For this review, use the dimensioned drawing (mm, ordinates from the lowest corner) and the shaded views. A direction names the side the tool comes from. Coordinates: 2 decimals unless noted, no trailing zeros. Order: outer loops, then holes, each group sorted by start corner. A loop starts at its lowest first (then second) coordinate and runs counter-clockwise, first axis right, second up. Notation, with made-up numbers: M -2,63 L 3,63 A24 cw 3,80 Z; hole C 70,50.25 d10. An arc over 180 degrees is marked long. Use CSV: the item, a comma, the result in double quotes.
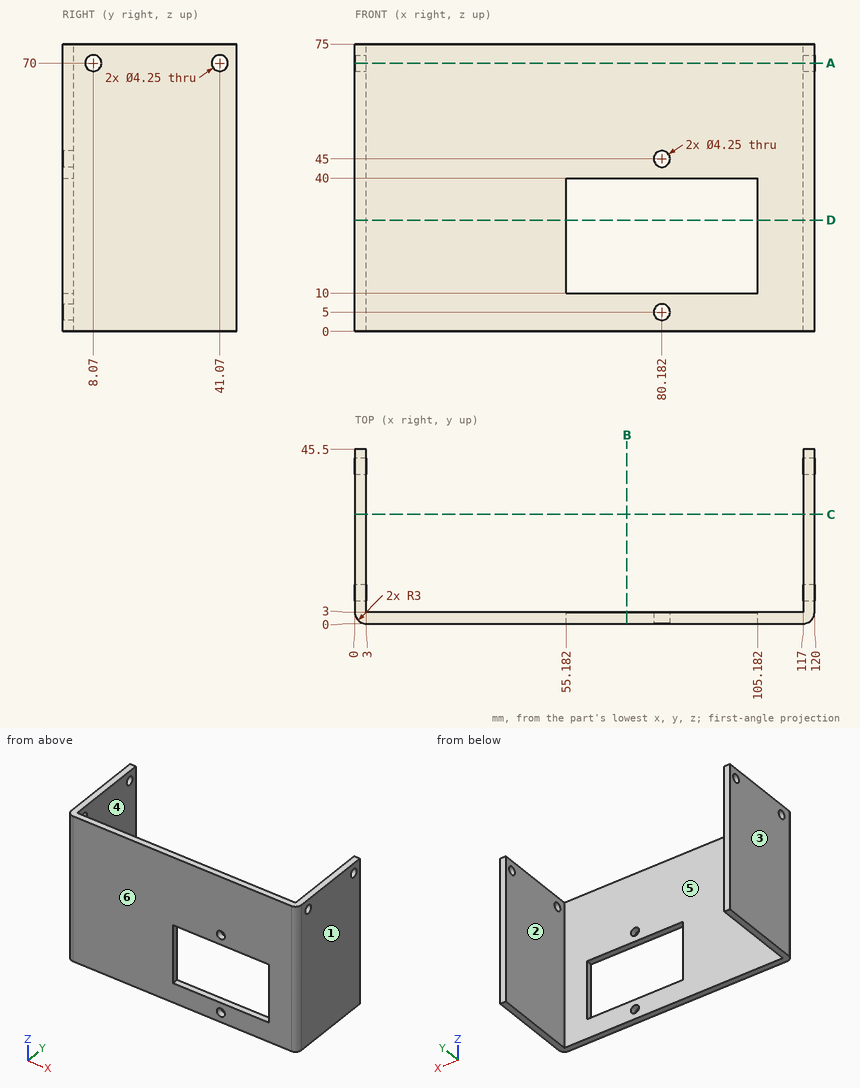
Item 1: Add section A-A on z = 70. State the section outline as (x, y) points (3 decimals), and give its area (3 significant figures).
Solutions:
outline,"M 0,3 A3 ccw 3,0 L 117,0 A3 ccw 120,3 L 120,5.945 L 117,5.945 L 117,3 L 3,3 L 3,5.945 L 0,5.945 Z; M 0,10.195 L 3,10.195 L 3,38.945 L 0,38.945 Z; M 0,43.195 L 3,43.195 L 3,45.5 L 0,45.5 Z; M 117,10.195 L 120,10.195 L 120,38.945 L 117,38.945 Z; M 117,43.195 L 120,43.195 L 120,45.5 L 117,45.5 Z"
area,"560 mm^2"
Item 2: To check wall thickness, follow line 1 along X through (y, z) = (43, 49.5); line 2 along Z through (x, y) = (70, 2); line 3 along Y through (x, z) = (14, 25.5). State the ranges of each line that lie inside material, in increasing order. Write a range as [from, to].
Solutions:
line 1,"[0, 3], [117, 120]"
line 2,"[0, 10], [40, 75]"
line 3,"[0, 3]"
Item 3: Clearance check with a flat-ended pin moving along its axis: pin 1 Ø3 at (x, z) = (63, 61.5) entering from +Y. State where the tip first meets the part, or that it passes through.
Solutions:
pin 1,"y = 3"
Item 4: For the marked faces 1 and 2, list the 3-axis set-ups (+Z, -Z, +X, -X, +Y, -Y) from which the entire face can be reached by the end or side of a thin tool; tool diameter is ignored.
Solutions:
face 1,"+Z, -Z, +X, +Y, -Y"
face 2,"+Z, -Z, +Y"
Item 5: Add section D-D on z = 29. State the section outline as (x, y) points, and give its area (3 significant figures).
Solutions:
outline,"M 0,3 A3 ccw 3,0 L 55.18,0 L 55.18,3 L 3,3 L 3,45.5 L 0,45.5 Z; M 105.18,0 L 117,0 A3 ccw 120,3 L 120,45.5 L 117,45.5 L 117,3 L 105.18,3 Z"
area,"461 mm^2"
Item 6: Add section C-C on y = 28.5. State the section outline as (x, z) points, and give its area (3 significant figures).
Solutions:
outline,"M 0,0 L 3,0 L 3,75 L 0,75 Z; M 117,0 L 120,0 L 120,75 L 117,75 Z"
area,"450 mm^2"
Item 7: Draft analysis for pull direction X (two halves, no side actions). For the marked faces 3, 4, 5 and 6, state which applies: released by +X, released by -X, zero draft, split by the parting line, or undercut.
Solutions:
face 3,"released by -X"
face 4,"undercut"
face 5,"undercut"
face 6,"zero draft"
Item 8: Add section B-B on x = 71. State the section outline as (y, z) points, and give its area (3 significant figures).
Solutions:
outline,"M 0,0 L 3,0 L 3,10 L 0,10 Z; M 0,40 L 3,40 L 3,75 L 0,75 Z"
area,"135 mm^2"
